```python
from build123d import *

# Parameters (mm, degrees)
BOSS_EXTRUDE1_DEPTH  = 10
M5_CLEARANCE_HOLE1_D = 5.5
GUSSET1_THICKNESS    = 4


with BuildPart() as part:
    # Sketch1 → Boss-Extrude1 (new, symmetric)
    with BuildSketch(Plane.XY):
        Polygon((0, 0), (0, 30), (6, 30), (6, 6), align=None)
    extrude(amount=BOSS_EXTRUDE1_DEPTH, both=True)

    # M5 Clearance Hole1 (through all)
    with Locations(Plane(origin=(6, 0, 0), x_dir=(0, 0, -1), z_dir=(1, 0, 0))):
        with Locations((0, 20)):
            Hole(M5_CLEARANCE_HOLE1_D / 2)

    # Mirror1: part across plane


with BuildPart() as part_1:
    add(part.part)
    add(part.part.mirror(Plane(origin=(0, 0, 10), x_dir=(0, 0, 1), z_dir=(0.7071067811865476, -0.7071067811865476, 0))))


with BuildPart() as body_2:
    # Gusset1: a gusset: a plate 4.0 thick in the corner of two members, its outline drawn in place
    gusset1_outline = Wire([Line((6, 6, -10), (6, 30, -10)), Line((6, 30, -10), (30, 6, -10)), Line((30, 6, -10), (6, 6, -10))])
    add(extrude(Face(gusset1_outline), amount=GUSSET1_THICKNESS, dir=(0, 0, 1)))


with BuildPart() as body_3:
    # Mirror3: mirrored copy
    add(body_2.part.mirror(Plane.XY))


with BuildPart() as part_2:
    add(part_1.part)

    # Combine1: union body 3, body 2
    add(body_3.part)
    add(body_2.part)


solid = part_2.part
```
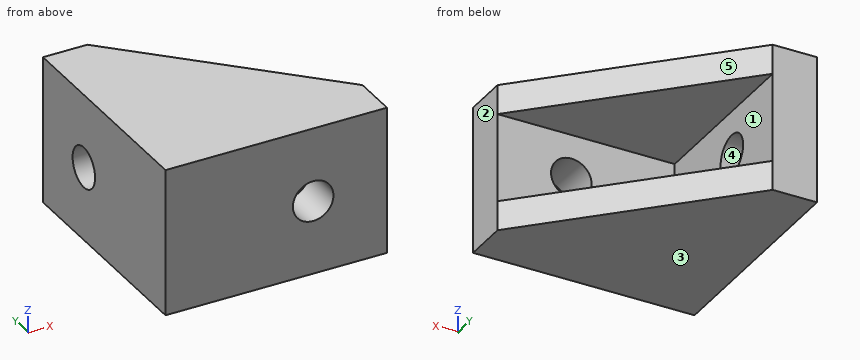
Could you check a few things on this model? Use its own coordinates, in mm. Face numbers are marked on the shaded views. A direction names the side the tool comes from. Give positions to 0.01 mm unless a question says otherwise; leave off trailing zeros. Loops run counter-clockwise (first coordinate to the right, second up) from the corner with the lowest first, then second, coordinate; pieces in that order, holes last. Notation, with made-up numbers: (63, 56.25) -> (69, 56.25) arc R13 ccw to (69, 68.25) -> close; hole circle Ø11 at (47.5, 78.25). An arc over 180 degrees is marked (long way). Put each result on its own line as item: value.
(1) Imagine slicing it at B-B on y = 20.5. Write out the boundary of the cut face in (x, z), plus the area to 3 significant figures.
Computed:
outline: (0, -10) -> (15.5, -10) -> (15.5, -6) -> (6, -6) -> (6, -2.7) -> (0, -2.7) -> close; (0, 2.7) -> (6, 2.7) -> (6, 6) -> (15.5, 6) -> (15.5, 10) -> (0, 10) -> close
area: 164 mm^2
(2) I'm going to push flat-ended pins straight in: pin 1 Ø5 at (y, z) = (16, 7.5) entering from +X; pin 2 Ø6 at (y, z) = (17.5, -8) entering from +X; pin 3 Ø9.5 at (y, z) = (18, -1) entering from +X; pin 4 Ø5 at (x, z) = (20, 0) entering from -Y. Where does each tip first touch, or does it pass through?
Computed:
pin 1: x = 22.5
pin 2: x = 21.5
pin 3: x = 6
pin 4: through
(3) For the marked faces 1 and 2, which set-ups out of +Z, -Z, +X, -X, +Y, -Y let a thin tool reach every point of the face, with its end or its side?
Computed:
face 1: +X, +Y
face 2: +Z, -Z, +X, +Y, -Y
(4) Please list where these lines run through material, in increasing order: probe 1 along Y at (x, z) = (3, 0); probe 2 along Z at (x, y) = (14.5, 9.5). Write a range as [from, to].
Computed:
probe 1: [0, 17.25], [22.75, 30]
probe 2: [-10, -6], [6, 10]
(5) Thinking about a two-plate mould opening in Z: for the marked faces 3, 4 and 5, which applies, pulls with the +Z half, pulls with the -Z half, needs draft (parallel to the pull), parting line crosses it, or undercut?
Computed:
face 3: pulls with the -Z half
face 4: undercut
face 5: needs draft
(6) Imagine slicing it at D-D on y = 11.5. Write out the boundary of the cut face in (x, z), plus the area to 3 significant figures.
Computed:
outline: (0, -10) -> (24.5, -10) -> (24.5, -6) -> (6, -6) -> (6, 6) -> (24.5, 6) -> (24.5, 10) -> (0, 10) -> close
area: 268 mm^2
(7) Imagine slicing it at C-C on x = 15.5. Write out the boundary of the cut face in (y, z), plus the area to 3 significant figures.
Computed:
outline: (0, -10) -> (20.5, -10) -> (20.5, -6) -> (6, -6) -> (6, 6) -> (20.5, 6) -> (20.5, 10) -> (0, 10) -> close
area: 236 mm^2
(8) Imagine slicing it at A-A on z = 0. Write out the boundary of the cut face in (x, y), plus the area to 3 significant figures.
Computed:
outline: (0, 0) -> (17.25, 0) -> (17.25, 6) -> (6, 6) -> (6, 17.25) -> (0, 17.25) -> close; (0, 22.75) -> (6, 22.75) -> (6, 30) -> (0, 30) -> close; (22.75, 0) -> (30, 0) -> (30, 6) -> (22.75, 6) -> close
area: 258 mm^2
